from build123d import *

# Parameters (mm, degrees)
SKETCH1_R           = 106.926704947
BOSS_EXTRUDE1_DEPTH = 40
DOME1_FACE_RADIUS   = 106.926704947
DOME1_HEIGHT        = 50
SKETCH2_W           = 5.57321272
SKETCH2_H           = 10.121090013
BOSS_EXTRUDE3_DEPTH = 0.1
SKETCH3_R           = 43.5
CUT_EXTRUDE2_DEPTH  = 250.43054033


with BuildPart() as part:
    # Sketch1 → Boss-Extrude1 (new body)
    with BuildSketch(Plane(origin=(0, 0, 0), x_dir=(1, 0, 0), z_dir=(0, 1, 0))):
        with Locations(Location((0, 0, 0), (0, 0, 270))):
            Circle(SKETCH1_R)
    extrude(amount=BOSS_EXTRUDE1_DEPTH)

    # Dome1: a dome of height H over a round flat face of radius A is a cap of a sphere of radius (A * A + H * H) / (2 * H)
    dome1_r = (DOME1_FACE_RADIUS * DOME1_FACE_RADIUS + DOME1_HEIGHT * DOME1_HEIGHT) / (2 * DOME1_HEIGHT)
    dome1_base = Plane((0, 40, 0), z_dir=(0, 1, 0))
    with Locations(dome1_base.offset(DOME1_HEIGHT - dome1_r)):
        dome1_ball = Sphere(dome1_r, mode=Mode.PRIVATE)
    add(split(dome1_ball, bisect_by=dome1_base, keep=Keep.TOP, mode=Mode.PRIVATE))

    # Sketch2 → Boss-Extrude3 (add)
    with BuildSketch(Plane(origin=(0, 0, 0), x_dir=(-1, 0, 0), z_dir=(0, -1, 0))):
        with Locations((-3.126868322, 94.609638257)):
            Rectangle(SKETCH2_W, SKETCH2_H)
    extrude(amount=BOSS_EXTRUDE3_DEPTH)

    # Sketch3 → Cut-Extrude2 (cut, through all)
    with BuildSketch(Plane(origin=(0, 0, -99.670183264), x_dir=(-1, 0, 0), z_dir=(0, 0, -1))):
        with Locations((2.431626064, 84.537651938)):
            Circle(SKETCH3_R)
    extrude(amount=-CUT_EXTRUDE2_DEPTH, mode=Mode.SUBTRACT)


solid = part.part
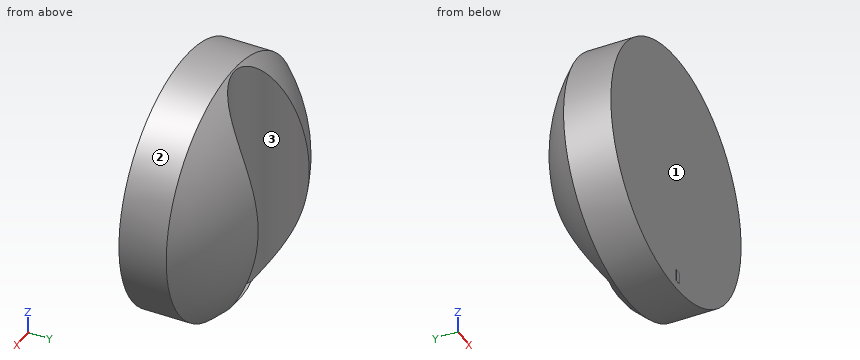
Part model, mm, in its own coordinate system. Face numbers are marked on the shaded views. Give positions to 0.01 mm unless a question says otherwise; leave off trailing zeros. Loops run counter-clockwise (first coordinate to the right, second up) from the corner with the lowest first, then second, coordinate; pieces in that order, holes last. Notation, with made-up numbers: M -5,79.25 L 27,79.25 A33 cw 27,112.25 Z; hole C 43.5,60 d11. An arc over 180 degrees is marked long. Put each result on its own line as item: value. Start each with the question number.
1) Pull direction X, two halves, no side cores. Call the marked faces 1, 2 and 3: +X half, -X half, draft (parallel to the pull), parting line (faces both ways), or undercut.
2) Flat gauge pins, fed straight in: pin 1 (12 mm diameter, centred on x = -33.5, y = 19.5, fed in from +Z); pin 2 (5 mm diameter, centred on x = -74.5, z = 60, fed in from -Y); pin 3 (8 mm diameter, centred on x = 83, y = 52.5, fed in from -Z). Where does each tip first touch, or does it go through?
3) Saw through at A-A (y = 9). List the corners of the cut face in (x, z), then the cut area to 3 significant figures.
4) Probe probe 1 along Y at (x, z) = (-1, -25); probe 2 along Y at (x, z) = (-1.5, -29); probe 3 along X at (y, z) = (67, 43). List the from-to ranges inside material, lowest first.
5) Saw through at D-D (y = 67). List the corners of the cut face in (x, z), then the cut area to 3 significant figures.
6) Saw through at B-B (x = 23.5). List the corners of the cut face in (y, z).
7) Saw through at C-C (z = -57). List the corners of the cut face in (x, y), then the cut area to 3 significant figures.
Numbers:
1. face 1: draft
1. face 2: parting line
1. face 3: undercut
2. pin 1: z = 103.33
2. pin 2: y = 0
2. pin 3: z = -56.48
3. outline: C 0,0 d213.85
3. area: 35,900 mm^2
4. probe 1: 0 to 41.06
4. probe 2: 0 to 41.05
4. probe 3: -63.49 to -42.24, 37.38 to 63.49
5. outline: M -42.24,-64 L -42.24,64 A76.68 ccw Z; M 37.38,-66.96 A76.68 ccw 37.38,66.96 Z
5. area: 6,840 mm^2
6. outline: M 0,-104.31 L 40,-104.31 A137.34 ccw 49.61,-95.24 L 49.61,95.24 A137.34 ccw 40,104.31 L 0,104.31 Z
7. outline: M -90.47,0 L 90.47,0 L 90.47,40 A127.14 ccw 39.11,71.64 A43.5 cw -43.48,70.14 A127.14 ccw -90.47,40 Z
7. area: 9,770 mm^2
